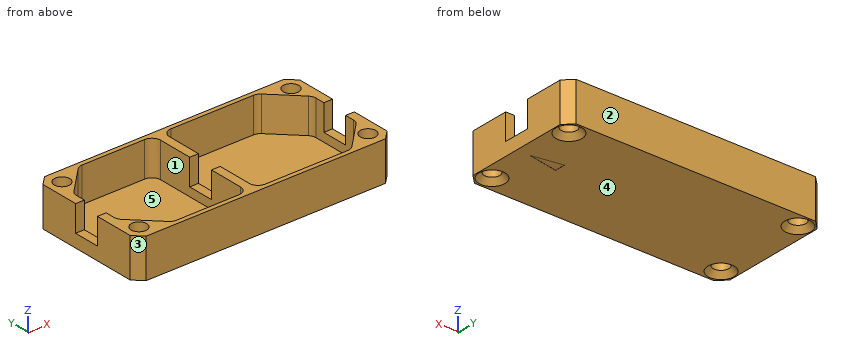
```python
from build123d import *

# Parameters (mm, degrees)
SKETCH_1_W              = 29.5
SKETCH_1_H              = 14
EXTRUDE_1_DEPTH         = 4.5
CUT_EXTRUDE_1_DEPTH     = 4
CHAMFER_1_SIZE          = 1
HOLE_WIZARD_M1_61_D     = 1.8
HOLE_WIZARD_M1_61_DEPTH = 14
HOLE_WIZARD_M1_61_TIP   = 0.540774557
FILLET_1_R              = 1
SKETCH_5_W              = 29.5
SKETCH_5_H              = 3
CUT_EXTRUDE_2_DEPTH     = 3
CHAMFER_2_SIZE          = 0.6
CUT_EXTRUDE_3_DEPTH     = 0.01


with BuildPart() as part:
    # Эскиз1 → Бобышка-Вытянуть1 (new body)
    with BuildSketch(Plane.XY):
        Rectangle(SKETCH_1_W, SKETCH_1_H)
    extrude(amount=EXTRUDE_1_DEPTH)

    # Эскиз2 → Вырез-Вытянуть1 (cut)
    with BuildSketch(Plane.XY.offset(4.5)):
        Polygon((-10.25, 6.5), (-1.65, 6.5), (-1.65, -6.5), (-10.25, -6.5), (-13.75, -3), (-13.75, 3), align=None)
        Polygon((-0.65, 6.5), (10.25, 6.5), (13.75, 3), (13.75, -3), (10.25, -6.5), (-0.65, -6.5), align=None)
    extrude(amount=-CUT_EXTRUDE_1_DEPTH, mode=Mode.SUBTRACT)

    # Фаска1
    chamfer_1_edges = [part.edges().sort_by_distance(p)[0] for p in [
        (14.75, -7, 2.25),
        (-14.75, -7, 2.25),
        (-14.75, 7, 2.25),
        (14.75, 7, 2.25),
    ]]
    chamfer(chamfer_1_edges, length=CHAMFER_1_SIZE)

    # Отверстие с зазором M1,61
    with Locations(Plane.XY.offset(4.5)):
        with Locations((-13.15, 5.3), (13.15, 5.3), (-13.15, -5.3), (13.15, -5.3)):
            Hole(HOLE_WIZARD_M1_61_D / 2, depth=HOLE_WIZARD_M1_61_DEPTH)
            with Locations((0, 0, -(HOLE_WIZARD_M1_61_DEPTH + HOLE_WIZARD_M1_61_TIP / 2))):  # 118° drill point
                Cone(0, HOLE_WIZARD_M1_61_D / 2, HOLE_WIZARD_M1_61_TIP, mode=Mode.SUBTRACT)

    # Скругление1
    fillet_1_edges = [part.edges().sort_by_distance(p)[0] for p in [
        (10.25, 6.5, 2.5),
        (13.75, 3, 2.5),
        (13.75, -3, 2.5),
        (10.25, -6.5, 2.5),
        (-0.65, -6.5, 2.5),
        (-0.65, 6.5, 2.5),
        (-13.75, 3, 2.5),
        (-10.25, 6.5, 2.5),
        (-1.65, 6.5, 2.5),
        (-1.65, -6.5, 2.5),
        (-10.25, -6.5, 2.5),
        (-13.75, -3, 2.5),
    ]]
    fillet(fillet_1_edges, radius=FILLET_1_R)

    # Эскиз5 → Вырез-Вытянуть2 (cut)
    with BuildSketch(Plane.XY.offset(4.5)):
        Rectangle(SKETCH_5_W, SKETCH_5_H)
    extrude(amount=-CUT_EXTRUDE_2_DEPTH, mode=Mode.SUBTRACT)

    # Фаска2
    chamfer_2_edges = [part.edges().sort_by_distance(p)[0] for p in [
        (14.05, -5.3, 0),
        (-12.25, -5.3, 0),
        (14.05, 5.3, 0),
        (-12.25, 5.3, 0),
    ]]
    chamfer(chamfer_2_edges, length=CHAMFER_2_SIZE)

    # Эскиз6 → Вырез-Вытянуть3 (cut)
    with BuildSketch(Plane(origin=(0, 0, 0), x_dir=(-1, 0, 0), z_dir=(0, 0, -1))):
        Polygon((-13.25, 0), (-9.75, 0.617144432), (-9.75, -0.617144432), align=None)
    extrude(amount=-CUT_EXTRUDE_3_DEPTH, mode=Mode.SUBTRACT)


solid = part.part
```
Work out the finished part from the listing and answer in its coordinate system (mm). Face numbers are marked on the shaded views. A direction names the side the tool comes from. Give positions to 0.01 mm unless a question says otherwise; leave off trailing zeros. Write each loop counter-clockwise with the first axis right and the second up, starting at its lowest first coordinate (ties: lowest second). Pieces come first, ordered by that corner, then holes. Notation, with made-up numbers: (17.25, 53) -> (22.25, 53) arc R6 ccw to (22.25, 64) -> close; hole circle Ø11 at (2, 82). An arc over 180 degrees is marked (long way). Write item = value, one per line.
Q1. Consider line 1 along X through (y, z) = (-2.5, 2.8); line 2 along Y through (x, z) = (9, 2.8). Determine where each line is inside the solid, lowest interval first.
Computed values:
line_1 = -14.75 to -13.75, -1.65 to -0.65, 13.75 to 14.75
line_2 = -7 to -6.5, 6.5 to 7
Q2. Section A-A on x = -13.15 is taken. Determine the outline of the cut face in (y, z), and give its area (3 significant figures).
Computed values:
outline = (-7, 0) -> (-6.8, 0) -> (-6.2, 0.6) -> (-6.2, 4.5) -> (-7, 4.5) -> close; (-4.4, 0.6) -> (-3.8, 0) -> (3.8, 0) -> (4.4, 0.6) -> (4.4, 4.5) -> (3.6, 4.5) -> (3.6, 0.5) -> (-3.6, 0.5) -> (-3.6, 4.5) -> (-4.4, 4.5) -> close; (6.2, 0.6) -> (6.8, 0) -> (7, 0) -> (7, 4.5) -> (6.2, 4.5) -> close
area = 17.3 mm^2
Q3. Section C-C on x = 7.25 is taken. Determine the outline of the cut face in (y, z), and give its area (3 significant figures).
Computed values:
outline = (-7, 0) -> (7, 0) -> (7, 4.5) -> (6.5, 4.5) -> (6.5, 0.5) -> (-6.5, 0.5) -> (-6.5, 4.5) -> (-7, 4.5) -> close
area = 11.0 mm^2
Q4. A tool of negligible diameter and unlimited length cuts with its end or side. For the marked faces 4 and 5, from which of +Z, -Z, +X, -X, +Y, -Y can it reach the whole face along a straight path? Write none if from no direction.
Computed values:
face_4 = -Z, +X, -X, +Y, -Y
face_5 = +Z
Q5. For a pull along X with two mould halves and no side action, classify the marked faces 1, 2 and 3 as pulls with the +X half, pulls with the -X half, needs draft (parallel to the pull), parting line crosses it, or undercut.
Computed values:
face_1 = undercut
face_2 = needs draft
face_3 = pulls with the -X half
Q6. Section B-B on z = 2.3 is taken. State how many separate pieces and enclosed holes the cut face has, and give its area (3 significant figures).
Computed values:
separate_pieces = 2
enclosed_holes = 4
area = 72.9 mm^2
Q7. Flat-ended cylindrical pins translate along their axes: pin 1 Ø0.8 at (x, y) = (-14.5, -0.5) entering from +Z; pin 2 Ø1.4 at (x, y) = (-13.15, -5.3) entering from +Z (3 decimals). Find the tip coordinate at first contact, or state that the pin passes through.
Computed values:
pin_1 = 1.5
pin_2 = through
